from build123d import *

# Parameters (mm, degrees)
SKETCH1_R                 = 1.625
BOSS_EXTRUDE1_DEPTH       = 4.7625
SKETCH6_R                 = 1.1
CUT_EXTRUDE3_DEPTH        = 5.7625
F_8_32_TAPPED_HOLE1_D     = 3.4544
F_8_32_TAPPED_HOLE1_DEPTH = 12.29
F_8_32_TAPPED_HOLE1_TIP   = 1.037806461


with BuildPart() as part:
    # Sketch1 → Boss-Extrude1 (new body)
    with BuildSketch(Plane(origin=(0, 0, 0), x_dir=(1, 0, 0), z_dir=(0, 1, 0))):
        with BuildLine():
            Line((-17, 6.25), (-17, 8))
            ThreePointArc((-17, 8), (-21, 12), (-25, 8))
            Line((-25, 8), (-25, 0))
            Line((-25, 0), (43, 0))
            Line((43, 0), (43, 6.25))
            Line((43, 6.25), (33, 6.25))
            Line((33, 6.25), (33, 12))
            ThreePointArc((33, 12), (29, 16), (25, 12))
            Line((25, 12), (25, 8.75))
            Line((25, 8.75), (-7, 8.75))
            Line((-7, 8.75), (-7, 6.25))
            Line((-7, 6.25), (-17, 6.25))
        make_face()
        with Locations((-21, 8)):
            Circle(SKETCH1_R, mode=Mode.SUBTRACT)
        with Locations((29, 12)):
            Circle(SKETCH1_R, mode=Mode.SUBTRACT)
    boss_extrude1 = extrude(amount=BOSS_EXTRUDE1_DEPTH)

    # Mirror1: Boss-Extrude1 across plane
    add(boss_extrude1.mirror(Plane.XY))

    # Sketch6 → Cut-Extrude3 (cut, through all)
    with BuildSketch(Plane(origin=(0, 4.7625, 0), x_dir=(1, 0, 0), z_dir=(0, 1, 0))):
        with Locations((5, -3)):
            Circle(SKETCH6_R)
        with Locations((-5, 3)):
            Circle(SKETCH6_R)
    extrude(amount=-CUT_EXTRUDE3_DEPTH, mode=Mode.SUBTRACT)

    # #8-32 Tapped Hole1
    with Locations(Plane(origin=(0, 4.7625, 0), x_dir=(-1, 0, 0), z_dir=(0, 1, 0))):
        with Locations((-34.85, 0)):
            Hole(F_8_32_TAPPED_HOLE1_D / 2, depth=F_8_32_TAPPED_HOLE1_DEPTH)
            with Locations((0, 0, -(F_8_32_TAPPED_HOLE1_DEPTH + F_8_32_TAPPED_HOLE1_TIP / 2))):  # 118° drill point
                Cone(0, F_8_32_TAPPED_HOLE1_D / 2, F_8_32_TAPPED_HOLE1_TIP, mode=Mode.SUBTRACT)


solid = part.part
Design review of the part built by this model. Coordinates are the model's own, in mm. A direction names the side the tool comes from. Round coordinates to 2 decimals unless told otherwise and drop trailing zeros. Write each loop counter-clockwise with the first axis right and the second up, starting at its lowest first coordinate (ties: lowest second). Pieces come first, ordered by that corner, then holes. Notation, with made-up numbers: (19.5, 19.5) - (54.5, 19.5) arc R16 cw to (54.5, 36.5) - close; hole circle Ø3 at (69.25, 83). An arc over 180 degrees is marked (long way). Return JSON: item names as keys, results as strings. Group by question number.
Item 1: We need section A-A on x = -21. Write out the cut boundary in (y, z) (1 decimal), and give its area (3 significant figures).
Item 2: We need section D-D on y = 2.65. Write out the cut boundary in (x, z) (3 decimals), and give its area (3 significant figures).
Item 3: Machinability: for faces 1 (the face through (-17, 2, -7)), 2 (the face through (33, 2, 9)), 3 (the face through (-12, 2, 6.25)), which of the approach directions +Z, -Z, +X, -X, +Y, -Y give a long, thin tool a straight path to every point of the face, cutting with its end or side? Answer none if there is none.
Item 4: Insertion check: P1, Ø1.4, axis at x = -10.5, y = 1.5, coming from the +Z side; P2, Ø2.5, axis at x = 13.5, y = 3, coming from the -Z side; P3, Ø0.9, axis at y = 3.5, z = -7, coming from the +X side; P4, Ø3.5, axis at x = -5, z = -3, coming from the +Y side. Each pin has a flat end and moves straight along its axis. Give the tip position at first contact, or say it passes through.
Item 5: We need section C-C on x = 34.85. Write out the cut boundary in (y, z).
Item 6: We need section B-B on z = 3. Write out the cut boundary in (x, y).
Item 7: For probe 1 along Z at (x, y) = (29, 1.05) (3 decimals); probe 2 along Z at (x, y) = (-21, 3.45) (3 decimals); probe 3 along Z at (x, y) = (-5, 2.45), list the stretches that pass through material, from the lowest coordinate up. Write a range as [from, to].
Item 8: The part is to be moulded in two halves that separate along Z. For faces 4 (the face through (-19.45, 2.35, 8.49)), 5 (the face through (33, 2, -9)), 6 (the face through (9, 2, -8.75)), 7 (the face through (-19.45, 2.35, -8.49)), say which applies: pulls with the +Z half, pulls with the -Z half, needs draft (parallel to the pull), parting line crosses it, or undercut.
Model answer:
{
 "1": {"outline": "(0, -12) - (4.8, -12) - (4.8, -9.6) - (0, -9.6) - close; (0, -6.4) - (4.8, -6.4) - (4.8, 6.4) - (0, 6.4) - close; (0, 9.6) - (4.8, 9.6) - (4.8, 12) - (0, 12) - close", "area": "83.3 mm²"},
 "2": {"outline": "(-25, -8) arc R4 ccw to (-17, -8) - (-17, -6.25) - (-7, -6.25) - (-7, -8.75) - (25, -8.75) - (25, -12) arc R4 ccw to (33, -12) - (33, -6.25) - (43, -6.25) - (43, 6.25) - (33, 6.25) - (33, 12) arc R4 ccw to (25, 12) - (25, 8.75) - (-7, 8.75) - (-7, 6.25) - (-17, 6.25) - (-17, 8) arc R4 ccw to (-25, 8) - close; hole circle Ø3.25 at (-21, -8); hole circle Ø3.25 at (-21, 8); hole circle Ø2.2 at (-5, -3); hole circle Ø2.2 at (5, 3); hole circle Ø3.25 at (29, -12); hole circle Ø3.25 at (29, 12); hole circle Ø3.454 at (34.85, 0)", "area": "1,180 mm²"},
 "3": {"face 1": "-Z, +Y, -Y", "face 2": "+Z, +X, +Y, -Y", "face 3": "+Z, +Y, -Y"},
 "4": {"P1": "stops at z = 6.25", "P2": "stops at z = -8.75", "P3": "stops at x = 33", "P4": "stops at y = 4.76"},
 "5": {"outline": "(0, -6.25) - (4.76, -6.25) - (4.76, -1.73) - (0, -1.73) - close; (0, 1.73) - (4.76, 1.73) - (4.76, 6.25) - (0, 6.25) - close"},
 "6": {"outline": "(-25, 0) - (3.9, 0) - (3.9, 4.76) - (-25, 4.76) - close; (6.1, 0) - (43, 0) - (43, 4.76) - (6.1, 4.76) - close"},
 "7": {"probe 1": "z = [-16, -13.625], [-10.375, 10.375], [13.625, 16]", "probe 2": "z = [-12, -9.625], [-6.375, 6.375], [9.625, 12]", "probe 3": "z = [-8.75, -4.1], [-1.9, 8.75]"},
 "8": {"face 4": "undercut", "face 5": "needs draft", "face 6": "pulls with the -Z half", "face 7": "undercut"}
}
